Job drawing, mm, ordinate dimensions from the low corner. One solid piece. A direction names the side the tool comes from. Coordinates: 2 decimals unless noted, no trailing zeros. Write each loop counter-clockwise with the first axis right and the second up, starting at its lowest first coordinate (ties: lowest second). Pieces come first, ordered by that corner, then holes. Notation, with made-up numbers: (67, -31) - (101, -31) arc R27 cw to (101, -12) - close; hole circle Ø3 at (83, -11.75). An arc over 180 degrees is marked (long way). Put each result on its own line as item: value. Start each with the question number.
1. Saw through at A-A, the plane x = 19.25. Write the cut outline in (y, z).
2. Drill centre lines: L1, parallel to Z at x = 12, y = 4; L2, parallel to X at y = 2.25, z = 4.5; L3, parallel to X at y = 4.75, z = 6. Where is each one in solid material? Low to high. Write a range as from..to.
3. Saw through at D-D, the plane x = 4. Write the cut outline in (y, z).
4. Drop flat-ended pins along their axis: P1, Ø2.5, axis at x = 19, y = 4.5, coming from the -Z side; P2, Ø1, axis at x = 15.5, z = 2, coming from the +Y side; P3, Ø1, axis at x = 11.5, z = 13.5, coming from the -Y side. Give the stop position or say it passes through.
5. Which spindle directions (+Z, -Z, +X, -X, +Y, -Y) get a long thin tool onto all of the face, cutting with end or side? Do the marked faces 1, 2, 3, 4 and 5. Say none if no direction does.
6. Pull direction X, two halves, no side cores. Call the marked faces 6 and 7: released by +X, released by -X, zero draft, split by the parting line, or undercut.
7. Saw through at B-B, the plane y = 1.25. Write the cut outline in (x, z) (1 decimal).
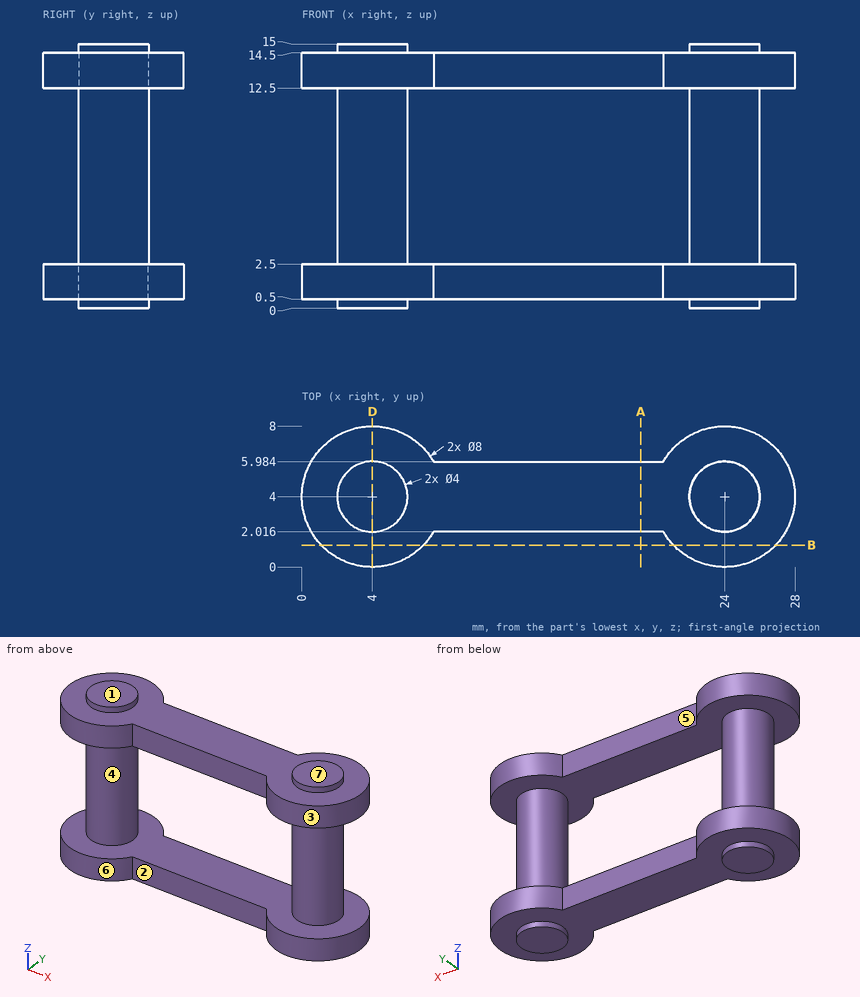
Final values:
1. outline: (2.02, 0.5) - (5.98, 0.5) - (5.98, 2.5) - (2.02, 2.5) - close; (2.02, 12.5) - (5.98, 12.5) - (5.98, 14.5) - (2.02, 14.5) - close
2. L1: z = 0.5..2.5, 12.5..14.5
2. L2: x = 3.03..4.97, 23.03..24.97
2. L3: x = 2.15..5.85, 22.15..25.85
3. outline: (0, 0.5) - (2, 0.5) - (2, 0) - (6, 0) - (6, 0.5) - (8, 0.5) - (8, 2.5) - (6, 2.5) - (6, 12.5) - (8, 12.5) - (8, 14.5) - (6, 14.5) - (6, 15) - (2, 15) - (2, 14.5) - (0, 14.5) - (0, 12.5) - (2, 12.5) - (2, 2.5) - (0, 2.5) - close
4. P1: stops at z = 0.5
4. P2: stops at y = 5.98
4. P3: stops at y = 2.02
5. face 1: +Z, +X, -X, +Y, -Y
5. face 2: +Z, -Z, -Y
5. face 3: +Z, -Z
5. face 4: none
5. face 5: +Z, -Z, +Y
6. face 6: undercut
6. face 7: zero draft
7. outline: (1.1, 0.5) - (6.9, 0.5) - (6.9, 2.5) - (1.1, 2.5) - close; (1.1, 12.5) - (6.9, 12.5) - (6.9, 14.5) - (1.1, 14.5) - close; (21.1, 0.5) - (26.9, 0.5) - (26.9, 2.5) - (21.1, 2.5) - close; (21.1, 12.5) - (26.9, 12.5) - (26.9, 14.5) - (21.1, 14.5) - close
